from build123d import *

# Parameters (mm, degrees)
SKETCH1_R              = 64
SKETCH1_R_2            = 60
RIM_DEPTH              = 28
SKETCH2_R              = 65.5
SKETCH2_R_2            = 63
INNER_BEAD_LIP_DEPTH   = 1.5
SKETCH3_R              = 65.5
SKETCH3_R_2            = 63
OUTER_BEAD_LIP_DEPTH   = 1.5
SKETCH4_R              = 61
WEB_DEPTH              = 7
SKETCH5_R              = 8
HUB_BOSS_DEPTH         = 24
SKETCH6_R              = 13
LIGHTENING_HOLES_DEPTH = 9
D_BORE_4MM_DEPTH       = 30
SKETCH8_R              = 1.3
GRUB_SCREW_M3_DEPTH    = 9
SKETCH9_R              = 1.9
GRUB_KEY_ACCESS_DEPTH  = 57.5


with BuildPart() as part:
    # Sketch1 → Rim (new body)
    with BuildSketch(Plane.XY):
        Circle(SKETCH1_R)
        Circle(SKETCH1_R_2, mode=Mode.SUBTRACT)
    extrude(amount=RIM_DEPTH)

    # Sketch2 → Inner_bead_lip (add)
    with BuildSketch(Plane.XY):
        Circle(SKETCH2_R)
        Circle(SKETCH2_R_2, mode=Mode.SUBTRACT)
    extrude(amount=INNER_BEAD_LIP_DEPTH)

    # Sketch3 → Outer_bead_lip (add)
    with BuildSketch(Plane.XY.offset(26.5)):
        Circle(SKETCH3_R)
        Circle(SKETCH3_R_2, mode=Mode.SUBTRACT)
    extrude(amount=OUTER_BEAD_LIP_DEPTH)

    # Sketch4 → Web (add)
    with BuildSketch(Plane.XY):
        Circle(SKETCH4_R)
    extrude(amount=WEB_DEPTH)

    # Sketch5 → Hub_boss (add)
    with BuildSketch(Plane.XY):
        Circle(SKETCH5_R)
    extrude(amount=HUB_BOSS_DEPTH)

    # Sketch6 → Lightening_holes (cut)
    with BuildSketch(Plane.XY.offset(-1)):
        with Locations((32.04293994, 18.5)):
            Circle(SKETCH6_R)
        with Locations((0, 37)):
            Circle(SKETCH6_R)
        with Locations((-32.04293994, 18.5)):
            Circle(SKETCH6_R)
        with Locations((-32.04293994, -18.5)):
            Circle(SKETCH6_R)
        with Locations((0, -37)):
            Circle(SKETCH6_R)
        with Locations((32.04293994, -18.5)):
            Circle(SKETCH6_R)
    extrude(amount=LIGHTENING_HOLES_DEPTH, mode=Mode.SUBTRACT)

    # Sketch7 → D_bore_4mm (cut)
    with BuildSketch(Plane.XY.offset(-1)):
        with BuildLine():
            Line((1.5, -1.397318861), (1.5, 1.397318861))
            ThreePointArc((1.5, 1.397318861), (-2.05, 0), (1.5, -1.397318861))
        make_face()
    extrude(amount=D_BORE_4MM_DEPTH, mode=Mode.SUBTRACT)

    # Sketch8 → Grub_screw_M3 (cut)
    with BuildSketch(Plane(origin=(0, 0, 0), x_dir=(0, 0, -1), z_dir=(1, 0, 0))):
        with Locations(Location((-3.6, 0, 0), (0, 0, 270))):
            Circle(SKETCH8_R)
    extrude(amount=GRUB_SCREW_M3_DEPTH, mode=Mode.SUBTRACT)

    # Sketch9 → Grub_key_access (cut)
    with BuildSketch(Plane(origin=(8.5, 0, 0), x_dir=(0, 0, -1), z_dir=(1, 0, 0))):
        with Locations((-3.6, 0)):
            Circle(SKETCH9_R)
    extrude(amount=GRUB_KEY_ACCESS_DEPTH, mode=Mode.SUBTRACT)


solid = part.part
Read the model definition and answer for the solid it produces. Units are mm, in the model's axes. A direction names the side the tool comes from. Round coordinates to 2 decimals unless told otherwise and drop trailing zeros. Write each loop counter-clockwise with the first axis right and the second up, starting at its lowest first coordinate (ties: lowest second). Pieces come first, ordered by that corner, then holes.
1. The part is cut by section A-A, the plane z = 21. Determine the outline of the cut face in (x, y), then the cut area to 3 significant figures.
2. Given pin 1 Ø1.5 at (x, z) = (-32, 9.5) entering from +Y; pin 2 Ø10 at (x, z) = (-9, 4) entering from +Y; pin 3 Ø1.9 at (y, z) = (0.5, 3.5) entering from +X, each flat-ended and moving along its own axis, determine where each tip first touches the part or whether it passes through.
3. The part is cut by section B-B, the plane x = 22.5. Determine the outline of the cut face in (y, z), then the cut area to 3 significant figures.
4. The part is cut by section C-C, the plane x = -34.5. Determine the outline of the cut face in (y, z) (3 decimals).
5. Which of the six approach directions +Z, -Z, +X, -X, +Y, -Y give full straight-line access (tool end or side, diameter ignored) to faces 5 (the face through (-59.94, 2.64, 17.35)), 6 (the face through (-13.87, -62.48, 13.82)), 7 (the face through (8.5, 0, 2))?
6. The part is cut by section D-D, the plane y = -43.5. Determine the outline of the cut face in (x, z).
7. Determine the mould class of faces 1 (the face through (63, -14, 1.5)), 2 (the face through (-1, -14, 0)), 3 (the face through (35.86, 0.08, 5.5)), 4 (the face through (-45.03, 19.07, 3.45)) for opening direction Z: pulls with the +Z half, pulls with the -Z half, needs draft (parallel to the pull), parting line crosses it, or undercut.
8. Straight lines are drawn through the part: L1, parallel to Y at x = 0, z = 2; L2, parallel to Y at x = -24, z = 5.75; L3, parallel to Y at x = -1, z = 21.5. For each, find the intervals that lie inside material, in ascending order.
Values:
1. outline: circle Ø128 at (0, 0); circle Ø16 at (0, 0); hole circle Ø120 at (0, 0); hole (1.5, -1.4) - (1.5, 1.4) arc R2.05 ccw (long way) to start
1. area: 1,750 mm2
2. pin 1: stops at y = 55.85
2. pin 2: stops at y = 65.33
2. pin 3: stops at x = 8.5
3. outline: (-61.51, 0) - (-27.33, 0) - (-27.33, 7) - (-55.62, 7) - (-55.62, 28) - (-61.51, 28) - (-61.51, 26.5) - (-59.91, 26.5) - (-59.91, 1.5) - (-61.51, 1.5) - close; (-9.67, 0) - (9.67, 0) - (9.67, 7) - (-9.67, 7) - close; (27.33, 0) - (61.51, 0) - (61.51, 1.5) - (59.91, 1.5) - (59.91, 26.5) - (61.51, 26.5) - (61.51, 28) - (55.62, 28) - (55.62, 7) - (27.33, 7) - close; hole circle Ø3.8 at (0, 3.6)
3. area: 770 mm2
4. outline: (-55.678, 0) - (-31.266, 0) - (-31.266, 7) - (-49.089, 7) - (-49.089, 28) - (-55.678, 28) - (-55.678, 26.5) - (-53.905, 26.5) - (-53.905, 1.5) - (-55.678, 1.5) - close; (-5.734, 0) - (5.734, 0) - (5.734, 7) - (-5.734, 7) - close; (31.266, 0) - (55.678, 0) - (55.678, 1.5) - (53.905, 1.5) - (53.905, 26.5) - (55.678, 26.5) - (55.678, 28) - (49.089, 28) - (49.089, 7) - (31.266, 7) - close
5. face 5: +Z
5. face 6: none
5. face 7: +X
6. outline: (-48.97, 0) - (-11.26, 0) - (-11.26, 7) - (-41.32, 7) - (-41.32, 28) - (-48.97, 28) - (-48.97, 26.5) - (-46.94, 26.5) - (-46.94, 1.5) - (-48.97, 1.5) - close; (11.26, 0) - (48.97, 0) - (48.97, 1.5) - (46.94, 1.5) - (46.94, 26.5) - (48.97, 26.5) - (48.97, 28) - (41.32, 28) - (41.32, 7) - (11.26, 7) - close
7. face 1: undercut
7. face 2: pulls with the -Z half
7. face 3: undercut
7. face 4: needs draft
8. L1: y = -64 to -50, -24 to -2.05, 2.05 to 24, 50 to 64
8. L2: y = -59.33 to -28.71, -8.29 to 8.29, 28.71 to 59.33
8. L3: y = -63.99 to -59.99, -7.94 to -1.79, 1.79 to 7.94, 59.99 to 63.99
